Check sheet for the modelled part. Datum: model origin and axes. Units: mm. A direction names the side the tool comes from. Round coordinates to 2 decimals unless told otherwise and drop trailing zeros. Loops run counter-clockwise (first coordinate to the right, second up) from the corner with the lowest first, then second, coordinate; pieces in that order, holes last. Notation, with made-up numbers: (81, 87.25) -> (90, 87.25) arc R7 ccw to (90, 98.25) -> close; hole circle Ø7 at (-5.5, 53.25). An arc over 180 degrees is marked (long way). Use one line per item in the form item = value. Start each with the question number.
(1) Material ranges on probe 1 along X at (y, z) = (-0.7, -1.5); probe 2 along X at (y, z) = (-4.4, -6); probe 3 along Z at (x, y) = (-37, -2.95), recorded low to high. Write a range as [from, to].
(2) Sectioned sample at B-B (x = 86). Record the cut outline in (y, z).
(3) Draft check along Z on faces 5 (the flat face through (36, -5.08, -19)), 6 (the flat face through (-21, -3, -10.004)), 7 (the flat face through (30, -2.54, -11)). Enter one of: released by +Z, released by -Z, zero draft, split by the parting line, or undercut.
(4) Go/stop test with flat-tipped pins: pin 1 (2.5 mm diameter, centred on x = 22.74, z = -5.1, fed in from -Y); pin 2 (8.5 mm diameter, centred on x = 32, z = 0.5, fed in from -Y); pin 3 (2.5 mm diameter, centred on y = -2, z = 8, fed in from +X); pin 4 (12 mm diameter, centred on x = 45.5, z = 2.5, fed in from +Y). Record where each tip stops, or that it passes through.
(5) Sectioned sample at A-A (y = -3.5). Record the cut outline in (x, z), and give its area (3 significant figures).
(6) Sectioned sample at C-C (z = -38.5). Record the cut outline in (x, y).
(7) Set-up check for faces 1 (the flat face through (81, -3, 0.156)), 2 (the flat face through (35.855, -3, -47)), 3 (the flat face through (19, -3, 12.856)), 4 (the flat face through (11.492, -3, -16)): record each of +Z, -Z, +X, -X, +Y, -Y from which the full face is reachable in a straight line by a thin tool's end or side.
from build123d import *

# Parameters (mm, degrees)
F0_W     = 63.5
F0_H     = 10.16
F0_W_2   = 14.2032613265
F0_H_2   = 12.7
F0_W_3   = 10.16
F0_W_4   = 13.7367386735
F0_H_3   = 46.99
F1_DEPTH = 5.08
F2_R     = 14
F3_DEPTH = 2.54
F4_R     = 1.45
F4_R_2   = 2.5
F5_DEPTH = 25.4


with BuildPart() as f1:
    # F0 (on Front) → F1 (new body)
    with BuildSketch(Plane.XZ):
        with Locations((-20.2580714928, -4.9235147662)):
            Rectangle(F0_W, F0_H)
        with Locations((18.5935591704, 6.5064852338)):
            Rectangle(F0_W_2, F0_H_2)
        with Locations((18.5935591704, -4.9235147662)):
            Rectangle(F0_W_2, F0_H)
        with Locations((30.7751898336, 6.5064852338)):
            Rectangle(F0_W_3, F0_H_2)
        with Locations((18.5935591704, -16.3535147662)):
            Rectangle(F0_W_2, F0_H_2)
        with Locations((42.7235591704, 6.5064852338)):
            Rectangle(F0_W_4, F0_H_2)
        with Locations((42.7235591704, -4.9235147662)):
            Rectangle(F0_W_4, F0_H)
        with Locations((30.7751898336, 36.3514852338)):
            Rectangle(F0_W_3, F0_H_3)
        with Locations((30.7751898336, -16.3535147662)):
            Rectangle(F0_W_3, F0_H_2)
        with Locations((81.3419285072, -4.9235147662)):
            Rectangle(F0_W, F0_H)
        with Locations((42.7235591704, -16.3535147662)):
            Rectangle(F0_W_4, F0_H_2)
        with Locations((30.7751898336, -46.1985147662)):
            Rectangle(F0_W_3, F0_H_3)
    extrude(amount=F1_DEPTH)

    # F2 (on face) → F3 (cut)
    with BuildSketch(Plane.XZ.offset(5.08)):
        with Locations((30.5391428791, -5.3559371654)):
            Circle(F2_R)
    extrude(amount=-F3_DEPTH, mode=Mode.SUBTRACT)

    # F4 (on face) → F5 (cut)
    with BuildSketch(Plane.XZ.offset(2.54)):
        with Locations((38.7418020368, -5.1013086922)):
            Circle(F4_R)
        with Locations((22.7418020368, -5.1013086922)):
            Circle(F4_R)
        with Locations((30.7751898336, -14.7041610032)):
            Circle(F4_R)
        with Locations((30.7751898336, 4.2958389968)):
            Circle(F4_R)
        with Locations((30.5391428791, -5.3559371654)):
            Circle(F4_R_2)
    extrude(amount=-F5_DEPTH, mode=Mode.SUBTRACT)


solid = f1.part
Checks:
q1.probe_1 = [-52.01, 25.7], [35.86, 113.09]
q1.probe_2 = [-52.01, 16.55], [44.52, 113.09]
q1.probe_3 = [-10, 0.16]
q2.outline = (-5.08, -10) -> (0, -10) -> (0, 0.16) -> (-5.08, 0.16) -> close
q3.face_5 = zero draft
q3.face_6 = released by -Z
q3.face_7 = undercut
q4.pin_1 = through
q4.pin_2 = -2.54
q4.pin_3 = 49.59
q4.pin_4 = 0
q5.outline = (-52.01, -10) -> (11.49, -10) -> (11.49, -22.7) -> (25.7, -22.7) -> (25.7, -69.69) -> (35.86, -69.69) -> (35.86, -22.7) -> (49.59, -22.7) -> (49.59, -10) -> (113.09, -10) -> (113.09, 0.16) -> (49.59, 0.16) -> (49.59, 12.86) -> (35.86, 12.86) -> (35.86, 59.85) -> (25.7, 59.85) -> (25.7, 12.86) -> (11.49, 12.86) -> (11.49, 0.16) -> (-52.01, 0.16) -> close; hole circle Ø28 at (30.54, -5.36)
q5.area = 2,980 mm2
q6.outline = (25.7, -5.08) -> (35.86, -5.08) -> (35.86, 0) -> (25.7, 0) -> close
q7.face_1 = +Z, +X, +Y, -Y
q7.face_2 = -Z, +X, +Y, -Y
q7.face_3 = +Z, -X, +Y, -Y
q7.face_4 = -Z, -X, +Y, -Y
